Geometry: final body of the model. Coordinates: model frame, mm. A direction names the side the tool comes from. Give positions to 0.01 mm unless a question says otherwise; leave off trailing zeros. Order: outer loops, then holes, each group sorted by start corner. A loop starts at its lowest first (then second) coordinate and runs counter-clockwise, first axis right, second up. Notation, with made-up numbers: (11.25, 1) - (47.25, 1) arc R34 cw to (47.25, 33) - close; hole circle Ø7 at (45.5, 19.25). An arc over 180 degrees is marked (long way). Use one line per item in the form item = value.
Autodesk Fusion 360 part; units mm, degrees
sketch "Sketch1" plane through (0, 0, 0) normal (0, 0, 1) x (1, 0, 0)
  line L0 (0, 0) -> (38.2, 0)
  line L1 (38.2, 0) -> (38.2, 66.3)
  line L2 (38.2, 66.3) -> (0, 66.3)
  line L3 (0, 66.3) -> (0, 0)
  dimension "d1" = 38.2
  dimension "d2" = 66.3
extrude "Extrude1" add sketch "Sketch1" along normal blind 1.3
sketch "Sketch2" plane through (0, 0, 1.3) normal (0, 0, 1) x (-1, 0, 0)
  line L0 (0, -66.3) -> (0, 0)
  line L1 (0, 0) -> (-38.2, 0)
  line L2 (-38.2, 0) -> (-38.2, -66.3)
  line L3 (-38.2, -66.3) -> (0, -66.3)
  line L4 (-0.6, -63.65) -> (-37.6, -63.65)
  line L5 (-37.6, -63.65) -> (-37.6, -2.65)
  line L6 (-37.6, -2.65) -> (-0.6, -2.65)
  line L7 (-0.6, -2.65) -> (-0.6, -63.65)
  line L8 (-37.6, -21.65) -> (-23.6, -21.65)
  line L9 (-23.6, -21.65) -> (-23.6, -44.65)
  line L10 (-23.6, -44.65) -> (-37.6, -44.65)
  line L11 (-37.6, -44.65) -> (-37.6, -21.65)
  line L12 (-0.6, -37.15) -> (-4, -37.15) construction
  circle A0 centre (-4, -37.15) radius 1.5
  dimension "d5" = 37
  dimension "d6" = 61
  dimension "d7" = 2.65
  dimension "d8" = 0.6
  dimension "d9" = 14
  dimension "d10" = 19
  dimension "d11" = 19
  dimension "d12" = 26.5
  dimension "d13" = 3
extrude "Extrude2" cut sketch "Sketch2" against normal blind 78 contours A0
extrude "Extrude3" cut sketch "Sketch2" against normal blind 2 contours L5 L8 L9 L10 L11
(1) Cut plane C-C on y = 30. Output: boundary loops of the cut face in (x, z).
Computed values:
outline = (0, 0) - (23.6, 0) - (23.6, 1.3) - (0, 1.3) - close; (37.6, 0) - (38.2, 0) - (38.2, 1.3) - (37.6, 1.3) - close
(2) Ray query, line 1 along X through (y, z) = (37.15, 0.3); line 2 along Y through (x, z) = (4, 0.6); line 3 along Y through (x, z) = (35, 0.15). Return the intervals inside material, ascending.
Computed values:
line_1 = 0 to 2.5, 5.5 to 23.6, 37.6 to 38.2
line_2 = 0 to 35.65, 38.65 to 66.3
line_3 = 0 to 21.65, 44.65 to 66.3
(3) Cut plane B-B on x = 26. Output: boundary loops of the cut face in (y, z).
Computed values:
outline = (0, 0) - (21.65, 0) - (21.65, 1.3) - (0, 1.3) - close; (44.65, 0) - (66.3, 0) - (66.3, 1.3) - (44.65, 1.3) - close
(4) Reachability of faces 4 (the face through (37.6, 33, 1)), 5 (the face through (19, 66.3, 1)) from +Z, -Z, +X, -X, +Y, -Y: full face, straight path, thin tool, end or side. Return the list, or none.
Computed values:
face_4 = +Z, -Z
face_5 = +Z, -Z, +X, -X, +Y
(5) Pull-direction query (X, two-part tool) for faces 1 (the face through (23.6, 33, 1)), 2 (the face through (19, 0, 1)), 3 (the face through (0, 34, 1)); classes: released by +X, released by -X, zero draft, split by the parting line, or undercut.
Computed values:
face_1 = undercut
face_2 = zero draft
face_3 = released by -X
(6) Cut plane D-D on z = 0.95. Output: boundary loops of the cut face in (x, y).
Computed values:
outline = (0, 0) - (38.2, 0) - (38.2, 66.3) - (0, 66.3) - close; hole circle Ø3 at (4, 37.15); hole (23.6, 21.65) - (37.6, 21.65) - (37.6, 44.65) - (23.6, 44.65) - close
(7) Cut plane A-A on y = 37.15. Output: boundary loops of the cut face in (x, z).
Computed values:
outline = (0, 0) - (2.5, 0) - (2.5, 1.3) - (0, 1.3) - close; (5.5, 0) - (23.6, 0) - (23.6, 1.3) - (5.5, 1.3) - close; (37.6, 0) - (38.2, 0) - (38.2, 1.3) - (37.6, 1.3) - close
